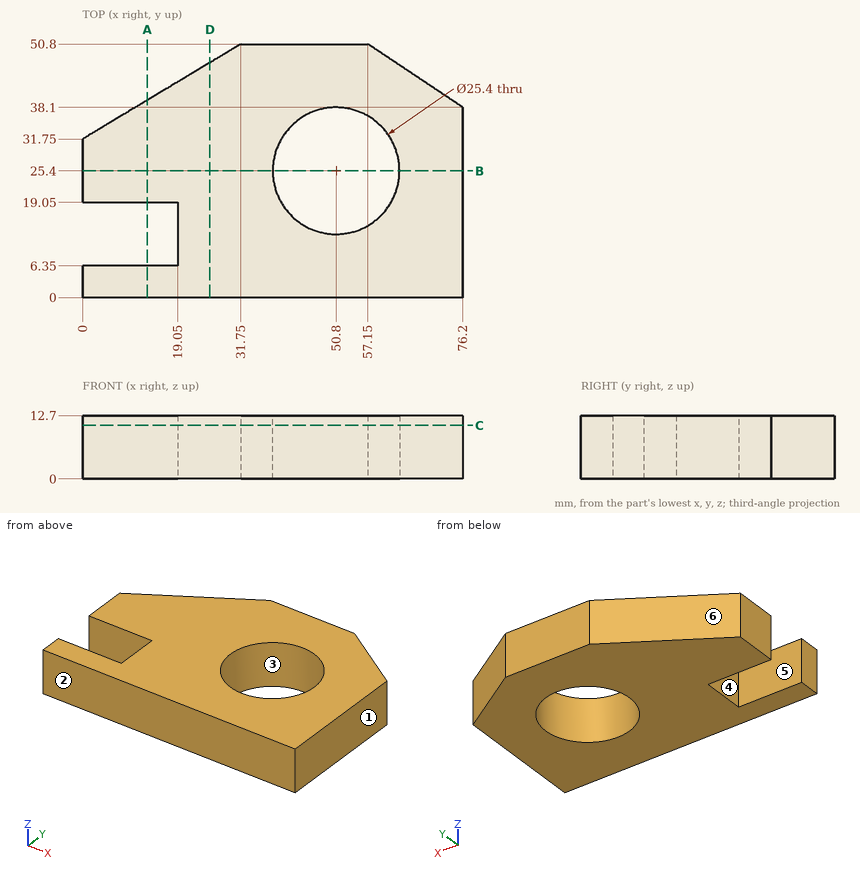
Could you check a few things on this drawing? It's one solid part, dimensions in mm from its lowest x, y, z. A direction names the side the tool comes from. Round coordinates to 2 decimals unless told otherwise and drop trailing zeros. Write each loop counter-clockwise with the first axis right and the second up, starting at its lowest first coordinate (ties: lowest second). Pieces come first, ordered by that corner, then holes.
Q1. If we section it at C-C on z = 10.75: Write out the boundary of the cut face in (x, y).
Q2. Which directions (+Z, -Z, +X, -X, +Y, -Y) give clear straight access to the entire face, cutting with the end or side of a thin tool? Please do the marked faces 5 and 6.
Q3. If we section it at D-D on x = 25.5: Write out the boundary of the cut face in (y, z).
Q4. Will this pin go through, and if not, where does the flat tip stop? P1, Ø1, axis at y = 8.5, z = 6.5, coming from the -X side.
Q5. If we section it at B-B on y = 25.4: Write out the boundary of the cut face in (x, z).
Q6. If we section it at A-A on x = 13: Write out the boundary of the cut face in (y, z).
Q7. Please list where these lines run through material, in increasing order: probe 1 along Y at (x, z) = (50.8, 8.5); probe 2 along X at (y, z) = (9, 1.25); probe 3 along X at (y, z) = (15, 5.75).
Q8. If we mould it in two halves opening along X, with no side actions, what happens to the marked faces 1, 2, 3 and 4? For each: +X half, -X half, draft (parallel to the pull), parting line (faces both ways), or undercut.
Answer below:
1. outline: (0, 0) - (76.2, 0) - (76.2, 38.1) - (57.15, 50.8) - (31.75, 50.8) - (0, 31.75) - (0, 19.05) - (19.05, 19.05) - (19.05, 6.35) - (0, 6.35) - close; hole circle Ø25.4 at (50.8, 25.4)
2. face 5: +Z, -Z, -X
2. face 6: +Z, -Z, -X, +Y
3. outline: (0, 0) - (47.05, 0) - (47.05, 12.7) - (0, 12.7) - close
4. P1: stops at x = 19.05
5. outline: (0, 0) - (38.1, 0) - (38.1, 12.7) - (0, 12.7) - close; (63.5, 0) - (76.2, 0) - (76.2, 12.7) - (63.5, 12.7) - close
6. outline: (0, 0) - (6.35, 0) - (6.35, 12.7) - (0, 12.7) - close; (19.05, 0) - (39.55, 0) - (39.55, 12.7) - (19.05, 12.7) - close
7. probe 1: y = 0 to 12.7, 38.1 to 50.8
7. probe 2: x = 19.05 to 76.2
7. probe 3: x = 19.05 to 43.51, 58.09 to 76.2
8. face 1: +X half
8. face 2: draft
8. face 3: undercut
8. face 4: -X half
